Source: CAD feature listing. Evaluate the final solid. Frame: model axes, mm. Face numbers are marked on the shaded views. A direction names the side the tool comes from. Give positions to 0.01 mm unless a question says otherwise; leave off trailing zeros. Loops run counter-clockwise (first coordinate to the right, second up) from the corner with the lowest first, then second, coordinate; pieces in that order, holes last. Notation, with made-up numbers: (-31, 19.5) -> (1, 19.5) arc R20 ccw to (1, 56.5) -> close; hole circle Ø6 at (37.25, 32.25). An arc over 180 degrees is marked (long way). Return JSON: item names as keys, results as strings. Group by question number.
(1) Cut plane A-A on x = 14. Return loops of the section in (y, z), then the cut area to 3 significant figures.
(2) Access query for the marked faces 1 and 2. Directions: +Z, -Z, +X, -X, +Y, -Y. A direction counts if a zero-diameter tool reaches every point of the face in a straight line with its end or side. Return the directions, or none.
(3) Pin query (flat end, axial travel): pin 1 (3 mm diameter, centred on x = 2.5, z = 1, fed in from -Y); pin 2 (1.5 mm diameter, centred on x = 6, y = 0, fed in from -Z); pin 3 (1.5 mm diameter, centred on x = 14.5, y = 0.5, fed in from +Z). Return the tip coordinate at first contact, or that it passes through.
(4) Ray query, line 1 (Z direction, x = 2.5, y = 0); line 2 (X direction, y = -1.7, z = 0.05); line 3 (Y direction, x = 5.5, z = 0.6). Return the intervals inside material, ascending. Write a range as from..to.
```python
from build123d import *

# Parameters (mm, degrees)
SKETCH3_W         = 0.79
SKETCH3_H         = 3.1
SKETCH4_W         = 0.395
SKETCH4_H         = 0.395
CIRPATTERN1_COUNT = 2
CIRPATTERN1_ANGLE = 90


with BuildPart() as part:
    # BodySke → Base-Revolve (revolve)
    with BuildSketch(Plane.XY):
        Polygon((0, 0), (0, 2.75), (0.45, 2.75), (1.7, 1.5), (16, 1.5), (16, 0), align=None)
    revolve(axis=Axis((-6.35, 0, 0), (1, 0, 0)))

    # Sketch3 → Cross section 0
    with BuildSketch(Plane.ZY):
        Rectangle(SKETCH3_W, SKETCH3_H)
    # Sketch4 → Cross section 1
    with BuildSketch(Plane.ZY.offset(-2.08)):
        Rectangle(SKETCH4_W, SKETCH4_H)
    cross = loft(mode=Mode.SUBTRACT)

    # CirPattern1: Cross ×2 about axis
    cirpattern1_axis = Axis((0, 0, 0), (1, 0, 0))
    for i in range(1, CIRPATTERN1_COUNT):
        add(cross.rotate(cirpattern1_axis, i * CIRPATTERN1_ANGLE / (CIRPATTERN1_COUNT - 1)), mode=Mode.SUBTRACT)


solid = part.part
```
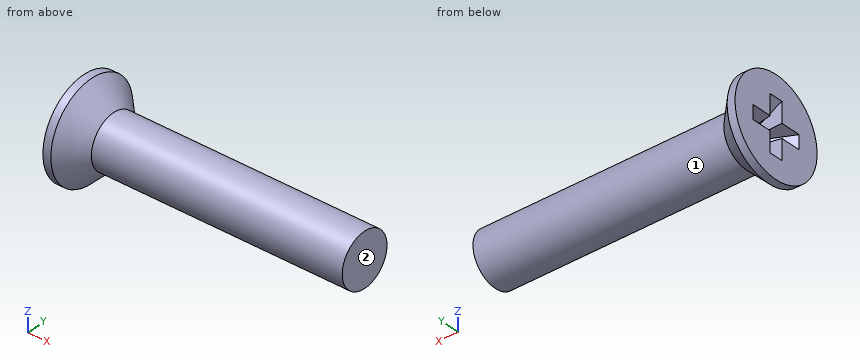
Answers:
{
 "1": {"outline": "circle Ø3 at (0, 0)", "area": "7.07 mm²"},
 "2": {"face 1": "+X", "face 2": "+Z, -Z, +X, +Y, -Y"},
 "3": {"pin 1": "y = -2.06", "pin 2": "z = -1.5", "pin 3": "z = 1.5"},
 "4": {"line 1": "-1.5..1.5", "line 2": "0..1.5", "line 3": "-1.37..1.37"}
}
